Can you work these out from the model? Positions are in its coordinate system, mm. Face numbers are marked on the shaded views. A direction names the side the tool comes from. Coordinates: 2 decimals unless noted, no trailing zeros. Put each result on its own line as item: value. Start each with the question number.
Item 1: Please list where these lines run through material, in increasing order: L1, parallel to Z at x = -6.5, y = 6; L2, parallel to Y at x = 0, z = -0.4; L3, parallel to Z at x = 2.5, y = 1. Write a range as from..to.
Item 2: Will these pins go through, and if not, where does the flat tip stop? P1, Ø4, axis at x = -11.5, y = -17, coming from the +Z side; P2, Ø0.8, axis at x = 0, y = 0, coming from the +Z side; P3, Ø8, axis at x = 4.5, y = -8.5, coming from the -Z side; P4, Ø1.5, axis at x = 11, z = -2, coming from the +Y side.
Item 3: For the marked faces 1 and 2, which set-ups out of +Z, -Z, +X, -X, +Y, -Y let a thin tool reach every point of the face, with its end or its side?
```python
from build123d import *

# Parameters (mm, degrees)
F2_R     = 0.5
F3_R     = 0.5
F4_R     = 0.5
F5_R     = 0.5
F6_R     = 0.5
F7_R     = 0.5
F8_DEPTH = 1


with BuildPart() as f1:
    # F0 (on Front) → F1 (revolve)
    with BuildSketch(Plane.XZ):
        Polygon((25, 0), (0, 0), (0, -6.4), (1.25, -6.4), (1.25, -2.4), (3.25, -2.4), (3.25, -1.6), (25, -1.6), align=None)
    revolve(axis=Axis((0, 0, 0.442708), (0, 0, -1)))

    # F2
    f2_edges = [f1.edges().sort_by_distance(p)[0] for p in [
        (-1.25, 0, -6.4),
    ]]
    fillet(f2_edges, radius=F2_R)

    # F3
    f3_edges = [f1.edges().sort_by_distance(p)[0] for p in [
        (-3.25, 0, -2.4),
    ]]
    fillet(f3_edges, radius=F3_R)

    # F4
    f4_edges = [f1.edges().sort_by_distance(p)[0] for p in [
        (-3.25, 0, -1.6),
    ]]
    fillet(f4_edges, radius=F4_R)

    # F5
    f5_edges = [f1.edges().sort_by_distance(p)[0] for p in [
        (-25, 0, -1.6),
    ]]
    fillet(f5_edges, radius=F5_R)

    # F6
    f6_edges = [f1.edges().sort_by_distance(p)[0] for p in [
        (-25, 0, 0),
    ]]
    fillet(f6_edges, radius=F6_R)

    # F7 (on face) → F8 (cut)
    with BuildSketch(Plane.XY):
        Circle(F7_R)
    extrude(amount=-F8_DEPTH, mode=Mode.SUBTRACT)


solid = f1.part
```
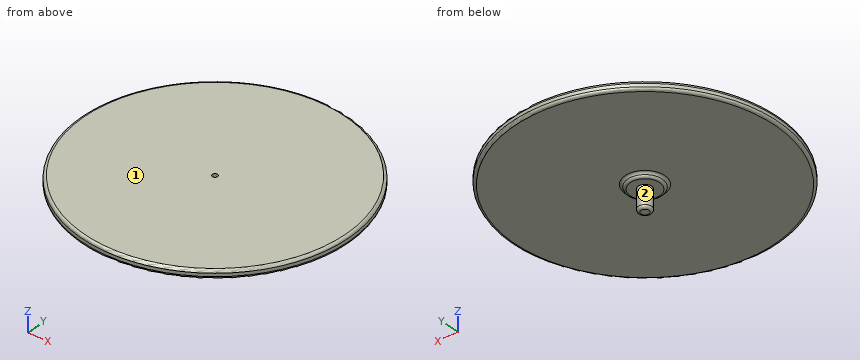
Solutions:
1. L1: -1.6..0
1. L2: -24.99..-0.5, 0.5..24.99
1. L3: -2.4..0
2. P1: z = 0
2. P2: z = -1
2. P3: z = -1.6
2. P4: y = 22.56
3. face 1: +Z, +X, -X, +Y, -Y
3. face 2: -Z
